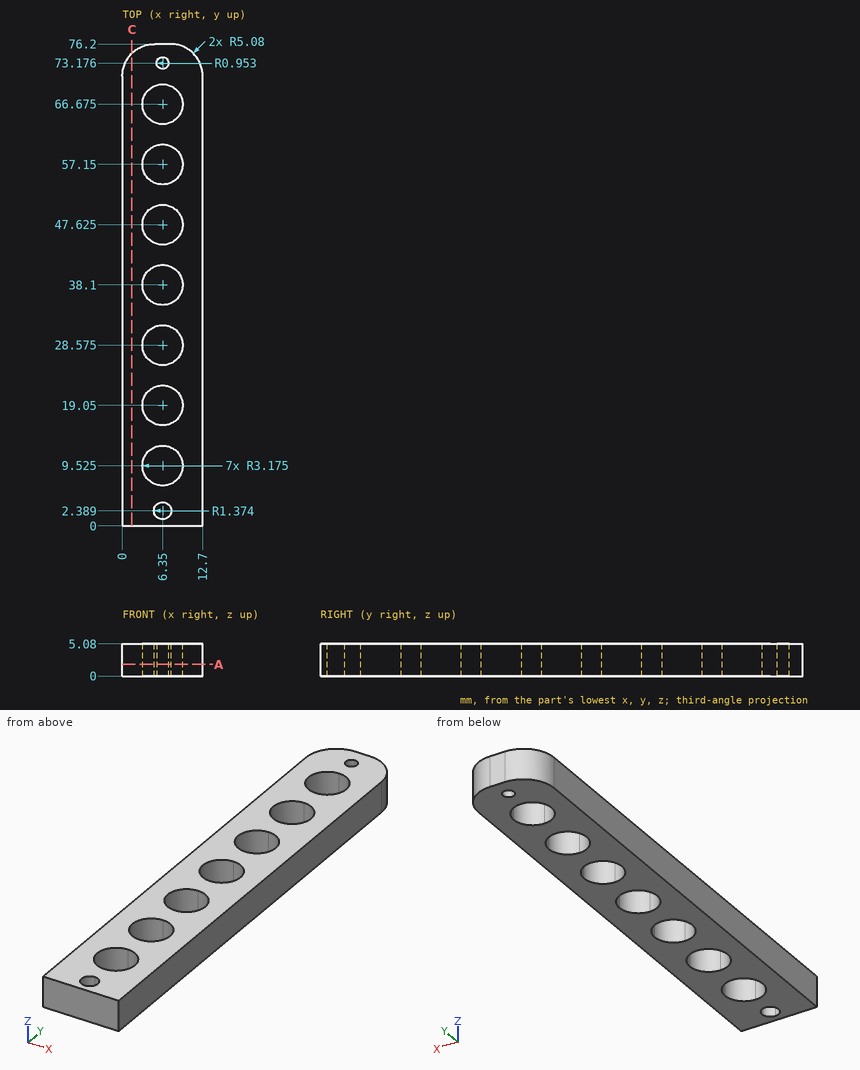
Here's the drawing with two shaded views (mm, measured from the low corner). I have some questions. Give positions to 0.01 mm unless a question says otherwise; leave off trailing zeros. Loops run counter-clockwise (first coordinate to the right, second up) from the corner with the lowest first, then second, coordinate; pieces in that order, holes last. Notation, with made-up numbers: (47, -37) - (103, -37) arc R8 ccw to (103, -32) - close; hole circle Ø6 at (-33, 14.5). An arc over 180 degrees is marked (long way). Return JSON: item names as keys, results as strings.
1. I want a section at A-A on z = 1.85. Give the number of separate pieces and of enclosed holes in the cut face.
Output values:
{"separate pieces": "1", "enclosed holes": "9"}
2. I'm going to push a flat-ended pin straight in: pin 1 Ø2 at (x, y) = (5.5, 8.5) entering from -Z. Where does the tip first touch, or does it pass through?
Output values:
{"pin 1": "passes through"}
3. If I drill on line 1 (X direction, y = 28.5, z = 3.15) (1 decimal); line 2 (X direction, y = 26.5, z = 1.35) (1 decimal); line 3 (Y direction, x = 2, z = 4.6), over which ranges is the centre line in solid material (lowest first)?
Output values:
{"line 1": "x = 0 to 3.2, 9.5 to 12.7", "line 2": "x = 0 to 3.9, 8.8 to 12.7", "line 3": "y = 0 to 75.16"}
4. I want a section at C-C on x = 1.5. Please give me the cut outline in (y, z) (1 decimal).
Output values:
{"outline": "(0, 0) - (74.7, 0) - (74.7, 5.1) - (0, 5.1) - close"}
